Check sheet for the modelled part. Datum: model origin and axes. Units: mm. A direction names the side the tool comes from. Give positions to 0.01 mm unless a question says otherwise; leave off trailing zeros. Loops run counter-clockwise (first coordinate to the right, second up) from the corner with the lowest first, then second, coordinate; pieces in that order, holes last. Notation, with made-up numbers: (53.25, 75.25) -> (92.25, 75.25) arc R23 ccw to (92.25, 111.25) -> close; hole circle Ø3 at (-9, 66). An arc over 180 degrees is marked (long way). Answer as CSV lines item,"result". Start each with the question number.
(1) Section check A-A on x = -4.25. Enter the section's corners in (y, z).
(2) Section check C-C on y = -3.75. Enter the section's corners in (x, z), plus the area to 3 significant figures.
(3) Access from +Z, -Z, +X, -X, +Y, -Y to the whole of each face (thin tool, end or side, straight path). Record for faces 4 (the face through (-4.277, -2.366, 1.972)), 5 (the face through (3.47, -3.43, 1.97)), 6 (the face through (-0.429, -2.818, 1.972)).
(4) Material ranges on line 1 (Y direction, x = -2, z = 1.95); line 2 (Y direction, x = 3, z = 2.3); line 3 (X direction, y = 2.25, z = 2.25), recorded low to high. Write a range as from..to.
(5) Release check for a two-part mould opening along Y. For faces 1 (the face through (2.225, -1.781, 1.972)), 2 (the face through (4.495, 1.823, 1.972)), 3 (the face through (-1, -8, 0)) record: pulls with the +Y half, pulls with the -Y half, needs draft (parallel to the pull), parting line crosses it, or undercut.
(6) Section check B-B on z = 2.1. Enter the section's corners in (x, y).
(7) Gauge pin test, flat end, axial feed: pin 1 Ø1 at (y, z) = (-9, 1.5) entering from -X. Record the tip position at first contact, or that the pin passes through.
(8) Section check D-D on y = -10.75. Enter the section's corners in (x, z), plus the area to 3 significant figures.
from build123d import *

# Parameters (mm, degrees)
BOSS_EXTRUDE1_DEPTH = 4


with BuildPart() as part:
    # Sketch1 → Boss-Extrude1 (new body)
    # profile 1 of 2: a face of its own
    with BuildSketch(Plane.XY):
        with BuildLine():
            ThreePointArc((-5.114216096, -0.273484418), (-5.236822192, 0.754506105), (-4.829006926, 1.70607506))
            Line((-4.829006926, 1.70607506), (-2.793952502, 4.29229885))
            ThreePointArc((-2.793952502, 4.29229885), (-1.964989642, 4.912474106), (-0.93699912, 5.035080203))
            Line((-0.93699912, 5.035080203), (2.320263594, 4.565783268))
            ThreePointArc((2.320263594, 4.565783268), (3.27183255, 4.157968002), (3.892007806, 3.329005142))
            Line((3.892007806, 3.329005142), (5.114216096, 0.273484418))
            ThreePointArc((5.114216096, 0.273484418), (5.236822192, -0.754506105), (4.829006926, -1.70607506))
            Line((4.829006926, -1.70607506), (2.079898318, -5.199745794))
            Line((2.079898318, -5.199745794), (-3.463162792, -4.401117677))
            Line((-3.463162792, -4.401117677), (-5.114216096, -0.273484418))
        make_face()
        Polygon((-2.035054424, -2.58622379), (1.22220829, -3.055520724), (3.257262714, -0.469296935), (2.035054424, 2.58622379), (-1.22220829, 3.055520724), (-3.257262714, 0.469296935), align=None, mode=Mode.SUBTRACT)
    # profile 2 of 2: a face of its own
    with BuildSketch(Plane.XY):
        with BuildLine():
            ThreePointArc((-3.967355061, -21.92537395), (-5.283579161, -21.143901064), (-5.66170537, -19.660605301))
            Line((-5.66170537, -19.660605301), (-3.463162792, -4.401117677))
            Line((-3.463162792, -4.401117677), (2.079898318, -5.199745794))
            Line((2.079898318, -5.199745794), (-0.11864426, -20.459233418))
            ThreePointArc((-0.11864426, -20.459233418), (-0.900117146, -21.775457517), (-2.383412909, -22.153583726))
            Line((-2.383412909, -22.153583726), (-3.967355061, -21.92537395))
        make_face()
    extrude(amount=BOSS_EXTRUDE1_DEPTH)


solid = part.part
Working result:
1,outline,"(-21.86, 0) -> (-9.86, 0) -> (-9.86, 4) -> (-21.86, 4) -> close; (-2.43, 0) -> (2.44, 0) -> (2.44, 4) -> (-2.43, 4) -> close"
2,outline,"(-3.72, 0) -> (3.22, 0) -> (3.22, 4) -> (-3.72, 4) -> close"
2,area,"27.8 mm^2"
3,face 4,"+Z, -Z, -X"
3,face 5,"+Z, -Z, +X, -Y"
3,face 6,"+Z, -Z"
4,line 1,"y = -22.17..-2.59, 2.07..4.9"
4,line 2,"y = -4.03..-0.8, 0.17..4.34"
4,line 3,"x = -4.4..-1.86, 2.17..4.32"
5,face 1,"undercut"
5,face 2,"pulls with the +Y half"
5,face 3,"needs draft"
6,outline,"(-5.66, -19.66) arc R2 ccw to (-3.97, -21.93) -> (-2.38, -22.15) arc R2 ccw to (-0.12, -20.46) -> (2.08, -5.2) -> (4.83, -1.71) arc R2 ccw to (5.11, 0.27) -> (3.89, 3.33) arc R2 ccw to (2.32, 4.57) -> (-0.94, 5.04) arc R2 ccw to (-2.79, 4.29) -> (-4.83, 1.71) arc R2 ccw to (-5.11, -0.27) -> (-3.46, -4.4) -> close; hole (-3.26, 0.47) -> (-2.04, -2.59) -> (1.22, -3.06) -> (3.26, -0.47) -> (2.04, 2.59) -> (-1.22, 3.06) -> close"
7,pin 1,"stops at x = -4.2"
8,outline,"(-4.38, 0) -> (1.28, 0) -> (1.28, 4) -> (-4.38, 4) -> close"
8,area,"22.6 mm^2"
